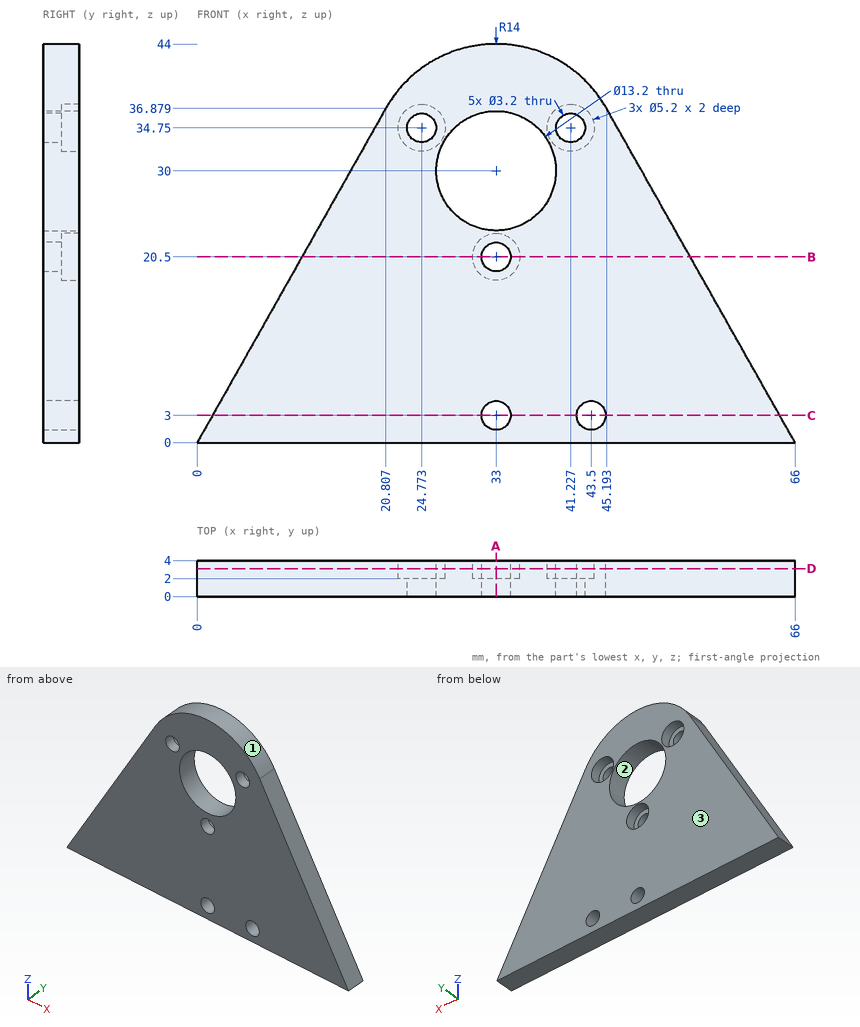
For this review, use the dimensioned drawing (mm, ordinates from the lowest corner) and the shaded views. Give positions to 0.01 mm unless a question says otherwise; leave off trailing zeros. Order: outer loops, then holes, each group sorted by start corner. A loop starts at its lowest first (then second) coordinate and runs counter-clockwise, first axis right, second up. Notation, with made-up numbers: (-13, -1) - (39, -1) arc R24 cw to (39, 19) - close; hole circle Ø1 at (57, 73). An arc over 180 degrees is marked (long way). Use CSV: the item, a comma, the result in double quotes. Start each with the question number.
Q1. The part is to be moulded in two halves that separate along Z. For the marked faces 1, 2 and 3, say which applies: +Z half, -Z half, draft (parallel to the pull), parting line (faces both ways), or undercut.
Q2. Clearance check with flat-ended pins moving along their axes: pin 1 Ø5 at (x, z) = (24.77, 34.75) entering from +Y; pin 2 Ø5.5 at (x, z) = (31.5, 20.5) entering from +Y; pin 3 Ø1.5 at (y, z) = (1.5, 23.5) entering from -X (1 decimal). State where each tip first meets the part, or that it passes through.
Q3. To check wall thickness, follow line 1 along X through (y, z) = (2.4, 3); line 2 along X through (y, z) = (2.9, 34.75) (1 decimal); line 3 along X through (y, z) = (2.35, 30) (1 decimal). State the ranges of each line that lie inside material, in increasing order. Write a range as [from, to].
Q4. We need section B-B, the plane z = 20.5. Write out the cut boundary in (x, y), and give its area (3 significant figures).
Q5. We need section C-C, the plane z = 3. Write out the cut boundary in (x, y).
Q6. We need section A-A, the plane x = 33. Write out the cut boundary in (y, z).
Q7. We need section D-D, the plane y = 3.1. Write out the cut boundary in (x, z).
Outcome:
1,face 1,"+Z half"
1,face 2,"undercut"
1,face 3,"draft"
2,pin 1,"stops at y = 2"
2,pin 2,"stops at y = 4"
2,pin 3,"stops at x = 12.8"
3,line 1,"x = [1.69, 31.4], [34.6, 41.9], [45.1, 64.31]"
3,line 2,"x = [19.6, 22.2], [27.4, 28.4], [37.6, 38.6], [43.8, 46.4]"
3,line 3,"x = [16.9, 26.4], [39.6, 49.1]"
4,outline,"(11.57, 0) - (31.4, 0) - (31.4, 2) - (30.4, 2) - (30.4, 4) - (11.57, 4) - close; (34.6, 0) - (54.43, 0) - (54.43, 4) - (35.6, 4) - (35.6, 2) - (34.6, 2) - close"
4,area,"155 mm^2"
5,outline,"(1.69, 0) - (31.4, 0) - (31.4, 4) - (1.69, 4) - close; (34.6, 0) - (41.9, 0) - (41.9, 4) - (34.6, 4) - close; (45.1, 0) - (64.31, 0) - (64.31, 4) - (45.1, 4) - close"
6,outline,"(0, 0) - (4, 0) - (4, 1.4) - (0, 1.4) - close; (0, 4.6) - (4, 4.6) - (4, 17.9) - (2, 17.9) - (2, 18.9) - (0, 18.9) - close; (0, 22.1) - (2, 22.1) - (2, 23.1) - (4, 23.1) - (4, 23.4) - (0, 23.4) - close; (0, 36.6) - (4, 36.6) - (4, 44) - (0, 44) - close"
7,outline,"(0, 0) - (66, 0) - (45.19, 36.88) arc R14 ccw to (20.81, 36.88) - close; hole circle Ø5.2 at (24.77, 34.75); hole circle Ø13.2 at (33, 30); hole circle Ø5.2 at (33, 20.5); hole circle Ø3.2 at (33, 3); hole circle Ø5.2 at (41.23, 34.75); hole circle Ø3.2 at (43.5, 3)"
